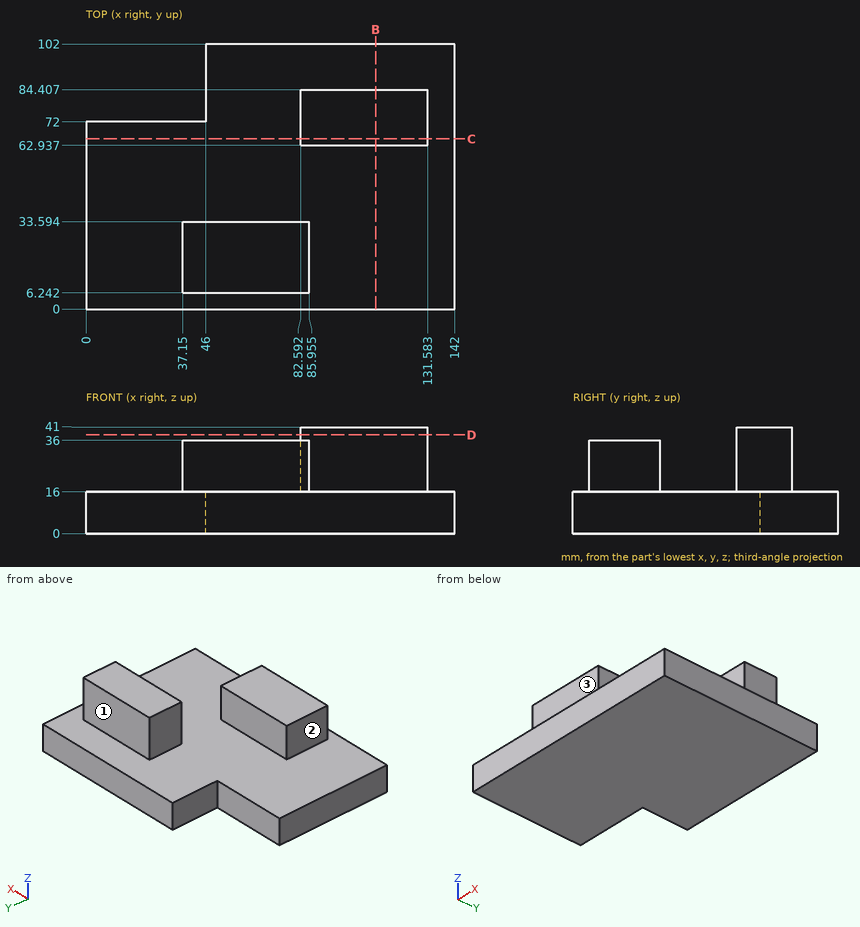
Input: dimensioned drawing with shaded views. Units: mm. Origin: part minimum x, y, z. A direction names the side the tool comes from. Coordinates: 2 decimals unless noted, no trailing zeros. Order: outer loops, then holes, each group sorted by start corner. A loop starts at its lowest first (then second) coordinate and runs counter-clockwise, first axis right, second up.
Item 1: Contact query for flat-ended pins moving along their axis: P1, Ø17.5, axis at y = 87, z = 7, coming from the -X side; P2, Ø6, axis at y = 17, z = 24.5, coming from the -X side; P3, Ø3, axis at x = 114, z = 25.5, coming from the +Y side; P4, Ø23.5, axis at y = 70, z = 25.5, coming from the +X side. Output: stop coordinate, or through.
Answer:
P1: stops at x = 46
P2: stops at x = 37.15
P3: stops at y = 84.41
P4: stops at x = 142
Item 2: Material intervals for line 1 along Y through (x, z) = (108, 20.5); line 2 along Y through (x, z) = (20, 8); line 3 along Z through (x, y) = (56.5, 86.5), sorted ascending.
Answer:
line 1: y = 62.94 to 84.41
line 2: y = 0 to 72
line 3: z = 0 to 16
Item 3: Section query C-C (y = 65.5). Output: boundary loops of the cut face in (x, z).
Answer:
outline: (0, 0) - (142, 0) - (142, 16) - (131.58, 16) - (131.58, 41) - (82.59, 41) - (82.59, 16) - (0, 16) - close
Item 4: Access query for the marked faces 1, 2 and 3. Directions: +Z, -Z, +X, -X, +Y, -Y. A direction counts if a zero-diameter tool reaches every point of the face in a straight line with its end or side. Return the directions, or none.
Answer:
face 1: +Z, +X, -X, +Y
face 2: +Z, -X, +Y, -Y
face 3: +Z, +X, -X, -Y
Item 5: Section query D-D (z = 38). Output: boundary loops of the cut face in (x, y), then the cut area to 3 significant figures.
Answer:
outline: (82.59, 62.94) - (131.58, 62.94) - (131.58, 84.41) - (82.59, 84.41) - close
area: 1,050 mm2
Item 6: Section query B-B (x = 111.5). Output: boundary loops of the cut face in (y, z), then the cut area to 3 significant figures.
Answer:
outline: (0, 0) - (102, 0) - (102, 16) - (84.41, 16) - (84.41, 41) - (62.94, 41) - (62.94, 16) - (0, 16) - close
area: 2,170 mm2
